Here's how the part is built. I have some questions about the finished solid (model axes, mm). A direction names the side the tool comes from. Coordinates: 2 decimals unless noted, no trailing zeros. Write each loop counter-clockwise with the first axis right and the second up, starting at its lowest first coordinate (ties: lowest second). Pieces come first, ordered by that corner, then holes. Notation, with made-up numbers: (34.25, 21) -> (47.25, 21) arc R20 ccw to (47.25, 57) -> close; hole circle Ø10 at (40.25, -24). An arc over 180 degrees is marked (long way). Put each result on its own line as item: value.
```python
from build123d import *

# Parameters (mm, degrees)
SKIZZE1_W                                    = 130
SKIZZE1_H                                    = 80
AUFSATZ_LINEAR_AUSTRAGEN1_DEPTH              = 6
F_2_4_2_4_DURCHMESSER_BOHRUNG1_D             = 2.4
F_2_4_2_4_DURCHMESSER_BOHRUNG1_DEPTH         = 10
F_2_4_2_4_DURCHMESSER_BOHRUNG1_CSINK_D       = 2.45
F_2_4_2_4_DURCHMESSER_BOHRUNG1_CSINK_ANGLE   = 90
F_2_4_2_4_DURCHMESSER_BOHRUNG1_TIP           = 0.721032743
STIRNSENKUNG_F_R_M2_FLACHKOPFSCHRAUB_2_COUNT = 2
STIRNSENKUNG_F_R_M2_FLACHKOPFSCHRAUB_2_PITCH = 48.918299235
STIRNSENKUNG_F_R_M2_FLACHKOPFSCHRAUB_3_COUNT = 2
STIRNSENKUNG_F_R_M2_FLACHKOPFSCHRAUB_3_PITCH = 74
STIRNSENKUNG_F_R_M2_FLACHKOPFSCHRAUB_4_COUNT = 2
STIRNSENKUNG_F_R_M2_FLACHKOPFSCHRAUB_4_PITCH = 95.268042911
STIRNSENKUNG_F_R_M2_FLACHKOPFSCHRAUB_5_COUNT = 2
STIRNSENKUNG_F_R_M2_FLACHKOPFSCHRAUB_5_PITCH = 99.161484458
STIRNSENKUNG_F_R_M2_FLACHKOPFSCHRAUB_6_COUNT = 2
STIRNSENKUNG_F_R_M2_FLACHKOPFSCHRAUB_6_PITCH = 60
SKIZZE8_R                                    = 1
SKIZZE8_W                                    = 30
SKIZZE8_H                                    = 15
SCHNITT_LINEAR_AUSTRAGEN1_DEPTH              = 6
VERRUNDUNG1_R                                = 3


with BuildPart() as part:
    # Skizze1 → Aufsatz-Linear austragen1 (new body)
    with BuildSketch(Plane(origin=(0, 0, 0), x_dir=(1, 0, 0), z_dir=(0, 1, 0))):
        with Locations((65, 40)):
            Rectangle(SKIZZE1_W, SKIZZE1_H)
    extrude(amount=AUFSATZ_LINEAR_AUSTRAGEN1_DEPTH)

    # Ø2.4 (2.4) Durchmesser Bohrung1
    with Locations(Plane(origin=(0, 6, 0), x_dir=(1, 0, 0), z_dir=(0, 1, 0))):
        with Locations((35, 77), (95, 77), (127, 40), (95, 3), (35, 3), (3, 40), (133.088689194, 32.803420387)):
            CounterSinkHole(F_2_4_2_4_DURCHMESSER_BOHRUNG1_D / 2, F_2_4_2_4_DURCHMESSER_BOHRUNG1_CSINK_D / 2, depth=F_2_4_2_4_DURCHMESSER_BOHRUNG1_DEPTH, counter_sink_angle=F_2_4_2_4_DURCHMESSER_BOHRUNG1_CSINK_ANGLE)
            with Locations((0, 0, -(F_2_4_2_4_DURCHMESSER_BOHRUNG1_DEPTH + F_2_4_2_4_DURCHMESSER_BOHRUNG1_TIP / 2))):  # 118° drill point
                Cone(0, F_2_4_2_4_DURCHMESSER_BOHRUNG1_D / 2, F_2_4_2_4_DURCHMESSER_BOHRUNG1_TIP, mode=Mode.SUBTRACT)

    # Skizze7 → Stirnsenkung für M2 Flachkopfschraube mit Schlitz1 (revolve, cut)
    with BuildSketch(Plane(origin=(95, 6, -3), x_dir=(0, 0, 1), z_dir=(1, 0, 0))):
        Polygon((0, 0), (0, 2.721032743), (1.2, 2), (1.2, 1.6), (2.5, 1.6), (2.5, 0.025), (2.525, 0), align=None)
    stirnsenkung_f_r_m2_flachkopfschraube_mi = revolve(axis=Axis((95, 12.35, -3), (0, -1, 0)), mode=Mode.SUBTRACT)

    # Stirnsenkung f_r M2 Flachkopfschraub 2: Stirnsenkung für M2 Flachkopfschraube mit Schlitz1 ×2
    with Locations(*[Vector(0.6541519329315842, 0, -0.7563631724521444) * (i * STIRNSENKUNG_F_R_M2_FLACHKOPFSCHRAUB_2_PITCH) for i in range(1, STIRNSENKUNG_F_R_M2_FLACHKOPFSCHRAUB_2_COUNT)]):
        add(stirnsenkung_f_r_m2_flachkopfschraube_mi, mode=Mode.SUBTRACT)

    # Stirnsenkung f_r M2 Flachkopfschraub 3: Stirnsenkung für M2 Flachkopfschraube mit Schlitz1 ×2
    with Locations(*[(0, 0, -i * STIRNSENKUNG_F_R_M2_FLACHKOPFSCHRAUB_3_PITCH) for i in range(1, STIRNSENKUNG_F_R_M2_FLACHKOPFSCHRAUB_3_COUNT)]):
        add(stirnsenkung_f_r_m2_flachkopfschraube_mi, mode=Mode.SUBTRACT)

    # Stirnsenkung f_r M2 Flachkopfschraub 4: Stirnsenkung für M2 Flachkopfschraube mit Schlitz1 ×2
    with Locations(*[Vector(-0.6298019584212194, 0, -0.7767557487195037) * (i * STIRNSENKUNG_F_R_M2_FLACHKOPFSCHRAUB_4_PITCH) for i in range(1, STIRNSENKUNG_F_R_M2_FLACHKOPFSCHRAUB_4_COUNT)]):
        add(stirnsenkung_f_r_m2_flachkopfschraube_mi, mode=Mode.SUBTRACT)

    # Stirnsenkung f_r M2 Flachkopfschraub 5: Stirnsenkung für M2 Flachkopfschraube mit Schlitz1 ×2
    with Locations(*[Vector(-0.9277795759357077, 0, -0.37312874249588235) * (i * STIRNSENKUNG_F_R_M2_FLACHKOPFSCHRAUB_5_PITCH) for i in range(1, STIRNSENKUNG_F_R_M2_FLACHKOPFSCHRAUB_5_COUNT)]):
        add(stirnsenkung_f_r_m2_flachkopfschraube_mi, mode=Mode.SUBTRACT)

    # Stirnsenkung f_r M2 Flachkopfschraub 6: Stirnsenkung für M2 Flachkopfschraube mit Schlitz1 ×2
    with Locations(*[(-i * STIRNSENKUNG_F_R_M2_FLACHKOPFSCHRAUB_6_PITCH, 0, 0) for i in range(1, STIRNSENKUNG_F_R_M2_FLACHKOPFSCHRAUB_6_COUNT)]):
        add(stirnsenkung_f_r_m2_flachkopfschraube_mi, mode=Mode.SUBTRACT)

    # Skizze8 → Schnitt-Linear austragen1 (cut)
    with BuildSketch(Plane(origin=(0, 6, 0), x_dir=(1, 0, 0), z_dir=(0, 1, 0))):
        with Locations(Location((47.606134621, 52.637382924, 0), (0, 0, 270))):
            Circle(SKIZZE8_R)
        with Locations(Location((58.356134621, 60.4477151, 0), (0, 0, 270))):
            Circle(SKIZZE8_R)
        with Locations(Location((71.643865379, 60.4477151, 0), (0, 0, 270))):
            Circle(SKIZZE8_R)
        with Locations(Location((82.393865379, 52.637382924, 0), (0, 0, 270))):
            Circle(SKIZZE8_R)
        with Locations(Location((86.5, 40, 0), (0, 0, 270))):
            Circle(SKIZZE8_R)
        with Locations(Location((82.393865379, 27.362617076, 0), (0, 0, 270))):
            Circle(SKIZZE8_R)
        with Locations(Location((71.643865379, 19.5522849, 0), (0, 0, 270))):
            Circle(SKIZZE8_R)
        with Locations(Location((58.356134621, 19.5522849, 0), (0, 0, 270))):
            Circle(SKIZZE8_R)
        with Locations(Location((47.606134621, 27.362617076, 0), (0, 0, 270))):
            Circle(SKIZZE8_R)
        with Locations(Location((43.5, 40, 0), (0, 0, 270))):
            Circle(SKIZZE8_R)
        with Locations((65, 40)):
            Rectangle(SKIZZE8_W, SKIZZE8_H)
    extrude(amount=-SCHNITT_LINEAR_AUSTRAGEN1_DEPTH, mode=Mode.SUBTRACT)

    # Verrundung1
    verrundung1_edges = [part.edges().sort_by_distance(p)[0] for p in [
        (50, 3, -47.5),
        (50, 3, -32.5),
        (80, 3, -32.5),
        (80, 3, -47.5),
    ]]
    fillet(verrundung1_edges, radius=VERRUNDUNG1_R)


solid = part.part
```
Item 1: Imagine slicing it at B-B on y = 3.35. State how many separate pieces and enclosed holes the cut face has, then the cut area to 3 significant figures.
Output:
separate pieces: 1
enclosed holes: 17
area: 9,900 mm²
Item 2: Imagine slicing it at A-A on x = 61. Write out the boundary of the cut face in (y, z).
Output:
outline: (0, -80) -> (6, -80) -> (6, -47.5) -> (0, -47.5) -> close; (0, -32.5) -> (6, -32.5) -> (6, 0) -> (0, 0) -> close
Item 3: Please list where these lines run through material, in increasing order: line 1 along X through (y, z) = (3.8, -52.5); line 2 along Z through (x, y) = (95, 5.4); line 3 along X through (y, z) = (3, -77). Write a range as from..to.
Output:
line 1: x = 0..46.62, 48.6..81.4, 83.38..130
line 2: z = -80..-79.5, -74.5..-5.5, -0.5..0
line 3: x = 0..33.8, 36.2..93.8, 96.2..130
Item 4: For P1, Ø2.5, axis at x = 96, z = -3.5, coming from the +Y side, with a flat end and sliding along its axis, tell me the tip position at first contact or that it passes through.
Output:
P1: stops at y = 4.4
Item 5: If we mould it in two halves opening along X, with no side actions, what happens to faces 1 (the cylindrical face through (124.52, 5.2, -40.33)), 2 (the flat face through (65, 3, -32.5)), 3 (the flat face through (130, 3, -39)), 4 (the flat face through (64, 6, -32))? For each: released by +X, released by -X, zero draft, split by the parting line, or undercut.
Output:
face 1: undercut
face 2: undercut
face 3: released by +X
face 4: zero draft
Item 6: Which directions (+Z, -Z, +X, -X, +Y, -Y) give clear straight access to the entire face, cutting with the end or side of a thin tool? Please do faces 5 (the flat face through (64, 3, -80)), 6 (the flat face through (50, 3, -40)), 7 (the flat face through (126, 4.4, -41)).
Output:
face 5: -Z, +X, -X, +Y, -Y
face 6: +Y, -Y
face 7: +Y
